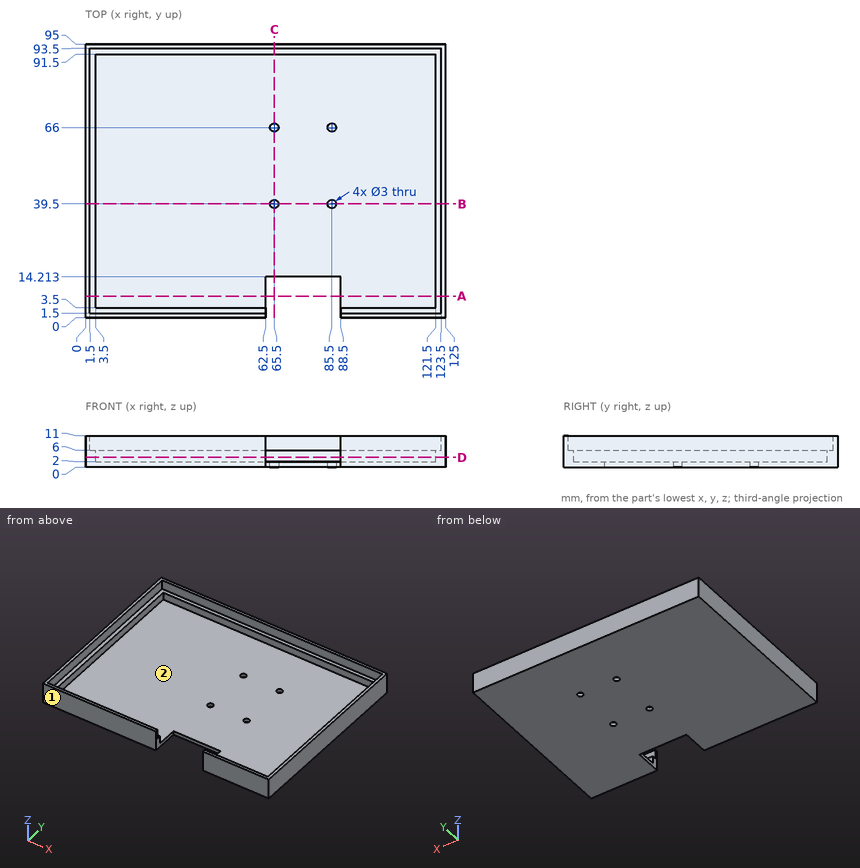
Print and shaded views of the part. All mm, measured from the part's lowest x, y and z. Give positions to 0.01 mm unless a question says otherwise; leave off trailing zeros. Order: outer loops, then holes, each group sorted by start corner. A loop starts at its lowest first (then second) coordinate and runs counter-clockwise, first axis right, second up. Notation, with made-up numbers: (-32.75, 67.5) -> (-22.75, 67.5) arc R11 ccw to (-22.75, 77.5) -> close; hole circle Ø9 at (-35, -36.75). An arc over 180 degrees is marked (long way). Use CSV: the item, a comma, the result in double quotes.
1. Band-saw the part on B-B, the plane y = 39.5. Give the cut face in (x, z).
Outcome:
outline,"(0, 0) -> (64, 0) -> (64, 2) -> (3.5, 2) -> (3.5, 6) -> (1.5, 6) -> (1.5, 11) -> (0, 11) -> close; (67, 0) -> (84, 0) -> (84, 2) -> (67, 2) -> close; (87, 0) -> (125, 0) -> (125, 11) -> (123.5, 11) -> (123.5, 6) -> (121.5, 6) -> (121.5, 2) -> (87, 2) -> close"
2. Mould opens along X. For the marked faces 1 and 2 say: +X half, -X half, draft (parallel to the pull), parting line (faces both ways), or undercut.
Outcome:
face 1,"draft"
face 2,"undercut"
3. Band-saw the part on D-D, the plane z = 3.5. Give the cut face in (x, y).
Outcome:
outline,"(0, 0) -> (62.5, 0) -> (62.5, 3.5) -> (3.5, 3.5) -> (3.5, 91.5) -> (121.5, 91.5) -> (121.5, 3.5) -> (88.5, 3.5) -> (88.5, 0) -> (125, 0) -> (125, 95) -> (0, 95) -> close"
4. Band-saw the part on C-C, the plane x = 65.5. Give the cut face in (y, z), then the cut area to 3 significant figures.
Outcome:
outline,"(14.21, 0) -> (38, 0) -> (38, 2) -> (14.21, 2) -> close; (41, 0) -> (64.5, 0) -> (64.5, 2) -> (41, 2) -> close; (67.5, 0) -> (95, 0) -> (95, 11) -> (93.5, 11) -> (93.5, 6) -> (91.5, 6) -> (91.5, 2) -> (67.5, 2) -> close"
area,"171 mm²"
5. Band-saw the part on A-A, the plane y = 7.5. Give the cut face in (x, z).
Outcome:
outline,"(0, 0) -> (62.5, 0) -> (62.5, 2) -> (3.5, 2) -> (3.5, 6) -> (1.5, 6) -> (1.5, 11) -> (0, 11) -> close; (88.5, 0) -> (125, 0) -> (125, 11) -> (123.5, 11) -> (123.5, 6) -> (121.5, 6) -> (121.5, 2) -> (88.5, 2) -> close"
6. Drill centre lines: line 1 along Y through (x, z) = (65.5, 1.1); line 2 along X through (y, z) = (5, 9.75); line 3 along X through (y, z) = (72, 5.25). Where is each one in solid material? Low to high. Write a range as from..to.
Outcome:
line 1,"14.21..38, 41..64.5, 67.5..95"
line 2,"0..1.5, 123.5..125"
line 3,"0..3.5, 121.5..125"
7. Drop flat-ended pins along their axis: pin 1 (1.8 mm diameter, centred on x = 65.5, y = 39.5, fed in from +Z); pin 2 (12 mm diameter, centred on x = 84.5, y = 42.5, fed in from +Z). Give the stop position or say it passes through.
Outcome:
pin 1,"through"
pin 2,"z = 2"
